from build123d import *

# Parameters (mm, degrees)
SKETCH1_R           = 4.5
BOSS_EXTRUDE1_DEPTH = 5
CUT_EXTRUDE1_DEPTH  = 10


with BuildPart() as part:
    # Sketch1 → Boss-Extrude1 (new body)
    with BuildSketch(Plane.XY):
        with BuildLine():
            Line((-60, 9), (60, 9))
            ThreePointArc((60, 9), (69, 0), (60, -9))
            Line((60, -9), (-60, -9))
            ThreePointArc((-60, -9), (-69, 0), (-60, 9))
        make_face()
        with Locations((-60, 0)):
            Circle(SKETCH1_R, mode=Mode.SUBTRACT)
        with Locations((60, 0)):
            Circle(SKETCH1_R, mode=Mode.SUBTRACT)
    extrude(amount=BOSS_EXTRUDE1_DEPTH)

    # Sketch2 → Cut-Extrude1 (cut)
    with BuildSketch(Plane.XY.offset(5)):
        with BuildLine():
            Line((-45, 4), (45, 4))
            ThreePointArc((45, 4), (49, 0), (45, -4))
            Line((45, -4), (-45, -4))
            ThreePointArc((-45, -4), (-49, 0), (-45, 4))
        make_face()
    extrude(amount=-CUT_EXTRUDE1_DEPTH, mode=Mode.SUBTRACT)


solid = part.part
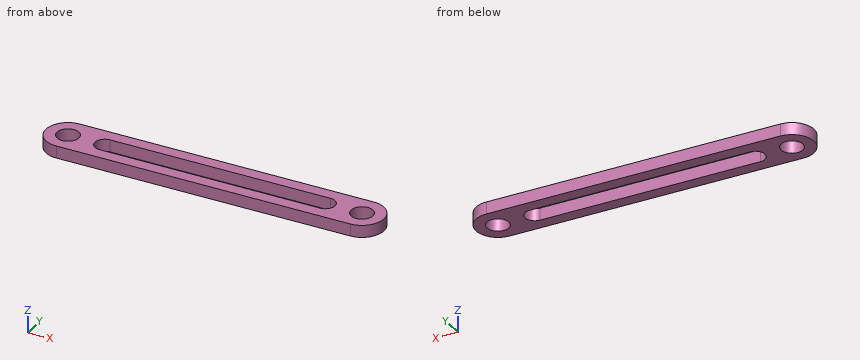
Read the model definition and answer for the solid it produces. Units are mm, in the model's axes. Coordinates: 2 decimals unless noted, no trailing zeros. Loops run counter-clockwise (first coordinate to the right, second up) from the corner with the lowest first, then second, coordinate; pieces in that order, holes last. Notation, with made-up numbers: (-37, 34.25) -> (8, 34.25) arc R6 ccw to (8, 39.25) -> close; hole circle Ø7 at (13, 78.25). An arc over 180 degrees is marked (long way). Answer in a Markdown table with one row per item.
Item 1: A cutting plane is placed at A-A on y = 0. Determine the outline of the cut face in (x, z).
Returned:
| item | result |
|---|---|
| outline | (-69, 0) -> (-64.5, 0) -> (-64.5, 5) -> (-69, 5) -> close; (-55.5, 0) -> (-49, 0) -> (-49, 5) -> (-55.5, 5) -> close; (49, 0) -> (55.5, 0) -> (55.5, 5) -> (49, 5) -> close; (64.5, 0) -> (69, 0) -> (69, 5) -> (64.5, 5) -> close |
Item 2: A cutting plane is placed at B-B on x = -26. Determine the outline of the cut face in (y, z), plus the area to 3 significant figures.
Returned:
| item | result |
|---|---|
| outline | (-9, 0) -> (-4, 0) -> (-4, 5) -> (-9, 5) -> close; (4, 0) -> (9, 0) -> (9, 5) -> (4, 5) -> close |
| area | 50.0 mm^2 |
Item 3: A cutting plane is placed at C-C on z = 1.6. Determine the outline of the cut face in (x, y).
Returned:
| item | result |
|---|---|
| outline | (-60, -9) -> (60, -9) arc R9 ccw to (60, 9) -> (-60, 9) arc R9 ccw to start; hole circle Ø9 at (-60, 0); hole (-45, -4) -> (45, -4) arc R4 ccw to (45, 4) -> (-45, 4) arc R4 ccw to start; hole circle Ø9 at (60, 0) |
Item 4: Each of these flat-tipped pins is pushed along its axis until it touches: P1, Ø7, axis at x = 60, y = 0, coming from the +Z side; P2, Ø3, axis at x = -50.5, y = -7, coming from the -Z side; P3, Ø1, axis at y = 4, z = 1.5, coming from the -X side. Where does it stop, or does it pass through?
Returned:
| item | result |
|---|---|
| P1 | passes through |
| P2 | stops at z = 0 |
| P3 | stops at x = -68.29 |
Item 5: A cutting plane is placed at D-D on y = 6.75. Determine the outline of the cut face in (x, z), plus the area to 3 significant figures.
Returned:
| item | result |
|---|---|
| outline | (-65.95, 0) -> (65.95, 0) -> (65.95, 5) -> (-65.95, 5) -> close |
| area | 660 mm^2 |
Item 6: Straight lines are drawn through the part: line 1 along X through (y, z) = (-1.75, 4); line 2 along Y through (x, z) = (-60, 1.2); line 3 along Y through (x, z) = (-28, 3.1). For each, find the intervals that lie inside material, in ascending order. Write a range as [from, to].
Returned:
| item | result |
|---|---|
| line 1 | x = [-68.83, -64.15], [-55.85, -48.6], [48.6, 55.85], [64.15, 68.83] |
| line 2 | y = [-9, -4.5], [4.5, 9] |
| line 3 | y = [-9, -4], [4, 9] |
